Autodesk Inventor part; units mm, degrees
ref_plane "YZ Plane" through (0, 0, 0) normal (1, 0, 0) x (0, 1, 0)
ref_plane "XZ Plane" through (0, 0, 0) normal (0, 1, 0) x (-1, 0, 0)
ref_plane "XY Plane" through (0, 0, 0) normal (0, 0, 1) x (1, 0, 0)
sketch "Szkic1" plane through (0, 0, 0) normal (0, 0, 1) x (1, 0, 0)
  line L0 (-9.1, 0) -> (9.1, 0)
  line L1 (0, -4.8) -> (0, 28.8)
  line L2 (-6.5, 24) -> (6.5, 24)
  line L3 (6.5, 24) -> (6.5, 0)
  line L4 (6.5, 0) -> (-6.5, 0)
  line L5 (-6.5, 0) -> (-6.5, 24)
  line L6 (0, 24) -> (0, 0)
  dimension "d0" = 13
  dimension "d1" = 24
extrude "Wyciągnięcie proste1" add sketch "Szkic1" against normal blind 17
sketch "Szkic2" plane through (6.5, 0, 0) normal (1, 0, 0) x (0, 0, -1)
  line L0 (17, 24) -> (17, 0)
  line L1 (17, 0) -> (3, 0)
  line L2 (3, 0) -> (3, 21)
  line L3 (3, 21) -> (17, 21)
  line L4 (17, 21) -> (17, 0)
  point P0 (0, 0)
  dimension "d4" = 14
  dimension "d5" = 21
extrude "Wyciągnięcie proste2" cut sketch "Szkic2" against normal blind 13
sketch "Szkic3" plane through (0, 0, 0) normal (0, 0, 1) x (1, 0, 0)
  line L0 (6.5, 24) -> (-6.5, 24)
  line L1 (-6.5, 0) -> (6.5, 0)
  point P0 (0, 0)
  point P1 (0, 16.3)
  point P2 (0, 3)
  dimension "d8" = 7.7
  dimension "d10" = 3
hole "Otwór1" at (0, 16.3, 0) at (0, 3, 0) direction (0, 0, -1) diameter 2.459 end through all
sketch "Szkic4" plane through (-6.5, 24, 0) normal (0, 1, 0) x (1, 0, 0)
  line L0 (13, 3) -> (0, 3)
  line L1 (0, 17) -> (13, 17)
  line L2 (6.5, 17) -> (6.5, 3)
  circle A0 centre (6.5, 12) radius 2.5
  line L3 (13, 0) -> (13, 17)
  line L4 (19, 12) -> (-6, 12)
  line L5 (0, 3) -> (-6, 3)
  line L6 (-6, 3) -> (-6, 17)
  line L7 (-6, 17) -> (0, 17)
  line L8 (0, 17) -> (0, 3)
  line L9 (13, 3) -> (19, 3)
  line L10 (19, 3) -> (19, 17)
  line L11 (19, 17) -> (13, 17)
  line L12 (13, 17) -> (13, 3)
  line L13 (-3.5, 3) -> (-3.5, 17)
  line L14 (0, 0) -> (0, 17)
  line L15 (0, 3) -> (0, 17)
  line L16 (16.5, 3) -> (16.5, 17)
  point P0 (6.5, 0)
  point P1 (0, 12)
  dimension "d18" = 5
  dimension "d20" = 5
  dimension "d21" = 6
  dimension "d22" = 6
  dimension "d23" = 3.5
extrude "Wyciągnięcie proste3" add sketch "Szkic4" against normal blind 3 contours L3 L4 L16 L9 | L3 L11 L16 L4 | L16 L4 L10 L9 | L5 L13 L4 L8 | L16 L11 L10 L4 | L5 L6 L4 L13 | L4 L13 L7 L8 | L4 L6 L7 L13
sketch "Szkic5" plane through (-6.5, 24, 0) normal (0, 1, 0) x (1, 0, 0)
  line L0 (13, 3) -> (0, 3)
  line L1 (6.5, 0) -> (6.5, 17)
  line L2 (-6, 17) -> (19, 17)
  line L3 (19, 17) -> (19, 3)
  line L4 (19, 12) -> (-6.0034, 12)
  line L5 (19, 3) -> (13, 3)
  line L6 (16.5, 3) -> (16.5, 17)
  line L7 (-3.5, 3) -> (-3.5, 17)
  circle A0 centre (6.4983, 12) radius 2.5
  dimension "d4" = 14
  dimension "d5" = 21
  dimension "d26" = 5
  dimension "d27" = 2.5
  dimension "d28" = 5
extrude "Wyciągnięcie proste4" cut sketch "Szkic5" against normal blind 3 contours A0 L4 L1 | L1 L4 A0 | L4 A0 L1 | L1 A0 L4
sketch "Szkic6" plane through (-6.5, 24, 0) normal (0, 1, 0) x (1, 0, 0)
  line L0 (6.5, 0) -> (6.5, 17)
  line L1 (-6, 17) -> (19, 17)
  line L2 (19, 17) -> (19, 3)
  line L3 (19, 12) -> (-5.9544, 12)
  line L4 (19, 3) -> (13, 3)
  line L5 (16.5, 3) -> (16.5, 17)
  line L6 (-3.5, 3) -> (-3.5, 17)
  point P0 (16.5, 12)
  point P1 (-3.5, 12)
  dimension "d31" = 5
  dimension "d32" = 2.5
hole "Otwór2" at (10, 24, -12) at (-10, 24, -12) direction (0, -1, 0) diameter 2.459 end through all
sketch "Szkic7" plane through (-6.5, 24, 0) normal (0, 1, 0) x (1, 0, 0)
  line L0 (19, 3) -> (13, 3)
  line L1 (19, 3) -> (21.5, 3)
  line L2 (21.5, 3) -> (21.5, 17)
  line L3 (21.5, 17) -> (19, 17)
  line L4 (19, 17) -> (19, 3)
  line L5 (-6, 3) -> (-6, 17)
  line L6 (-6, 3) -> (-8.5, 3)
  line L7 (-8.5, 3) -> (-8.5, 17)
  line L8 (-8.5, 17) -> (-6, 17)
  line L9 (-6, 17) -> (-6, 3)
  point P0 (6.5, 0)
  dimension "d40" = 2.5
  dimension "d41" = 2.5
extrude "Wyciągnięcie proste5" add sketch "Szkic7" against normal blind 3
properties part number "adapter" material "Stal nierdzewna 440C"
Design review of the part built by this model. Coordinates are the model's own, in mm. A direction names the side the tool comes from. Coordinates: 2 decimals unless noted, no trailing zeros. Loops run counter-clockwise (first coordinate to the right, second up) from the corner with the lowest first, then second, coordinate; pieces in that order, holes last.
Item 1: Add section D-D (z = -15.5). Write out the cut boundary in (x, y).
Completed:
outline: (-15, 21) - (15, 21) - (15, 24) - (-15, 24) - close
Item 2: Add section C-C (x = -10). Write out the cut boundary in (y, z), and give its area (3 significant figures).
Completed:
outline: (21, -17) - (24, -17) - (24, -13.23) - (21, -13.23) - close; (21, -10.77) - (24, -10.77) - (24, -3) - (21, -3) - close
area: 34.6 mm2
Item 3: Clearance check with flat-ended pins moving along their axes: pin 1 (4 mm diameter, centred on x = 0.5, y = 14.5, fed in from -Z); pin 2 (4 mm diameter, centred on x = 3.5, z = -13.5, fed in from -Y); pin 3 (1.5 mm diameter, centred on y = 15.5, z = -1.5, fed in from +X). State where each tip first meets the part, or that it passes through.
Completed:
pin 1: stops at z = -3
pin 2: stops at y = 21
pin 3: stops at x = 6.5
Item 4: For faces 1 (the flat face through (-11, 23, -3)), 2 (the flat face through (0, 21, -9)), 3 (the flat face through (-15, 23, -10)), list the 3-axis set-ups (+Z, -Z, +X, -X, +Y, -Y) from which the entire face can be reached by the end or side of a thin tool; tool diameter is ignored.
Completed:
face 1: +Z, -X, +Y, -Y
face 2: -Z, +X, -X, -Y
face 3: +Z, -Z, -X, +Y, -Y
Item 5: Wall thickness on L1, parallel to Y at x = 0, z = -2.3; L2, parallel to X at y = 22.2, z = -12; L3, parallel to Z at x = 10, y = 22.1: over which ranges is each line inside the solid? List them lowest first.
Completed:
L1: y = 0 to 1.77, 4.23 to 15.07, 17.53 to 24
L2: x = -15 to -11.23, -8.77 to -2.5, 2.5 to 8.77, 11.23 to 15
L3: z = -17 to -13.23, -10.77 to -3
Item 6: Draft analysis for pull direction Z (two halves, no side actions). For faces 4 (the cylindrical face through (-10.369, 22.479, -10.827)), 5 (the cylindrical face through (-0.54, 22.52, -9.56)), 6 (the flat face through (11, 23, -3)), 7 (the flat face through (15, 23, -10)), state which applies: pulls with the +Z half, pulls with the -Z half, needs draft (parallel to the pull), parting line crosses it, or undercut.
Completed:
face 4: undercut
face 5: undercut
face 6: pulls with the +Z half
face 7: needs draft
Item 7: Add section A-A (y = 16.3). Write out the cut boundary in (x, z).
Completed:
outline: (-6.5, -3) - (-1.23, -3) - (-1.23, 0) - (-6.5, 0) - close; (1.23, -3) - (6.5, -3) - (6.5, 0) - (1.23, 0) - close
Item 8: Add section B-B (x = 0). Write out the cut boundary in (y, z).
Completed:
outline: (0, -3) - (1.77, -3) - (1.77, 0) - (0, 0) - close; (4.23, -3) - (15.07, -3) - (15.07, 0) - (4.23, 0) - close; (17.53, -3) - (21, -3) - (21, -9.5) - (24, -9.5) - (24, 0) - (17.53, 0) - close; (21, -17) - (24, -17) - (24, -14.5) - (21, -14.5) - close
